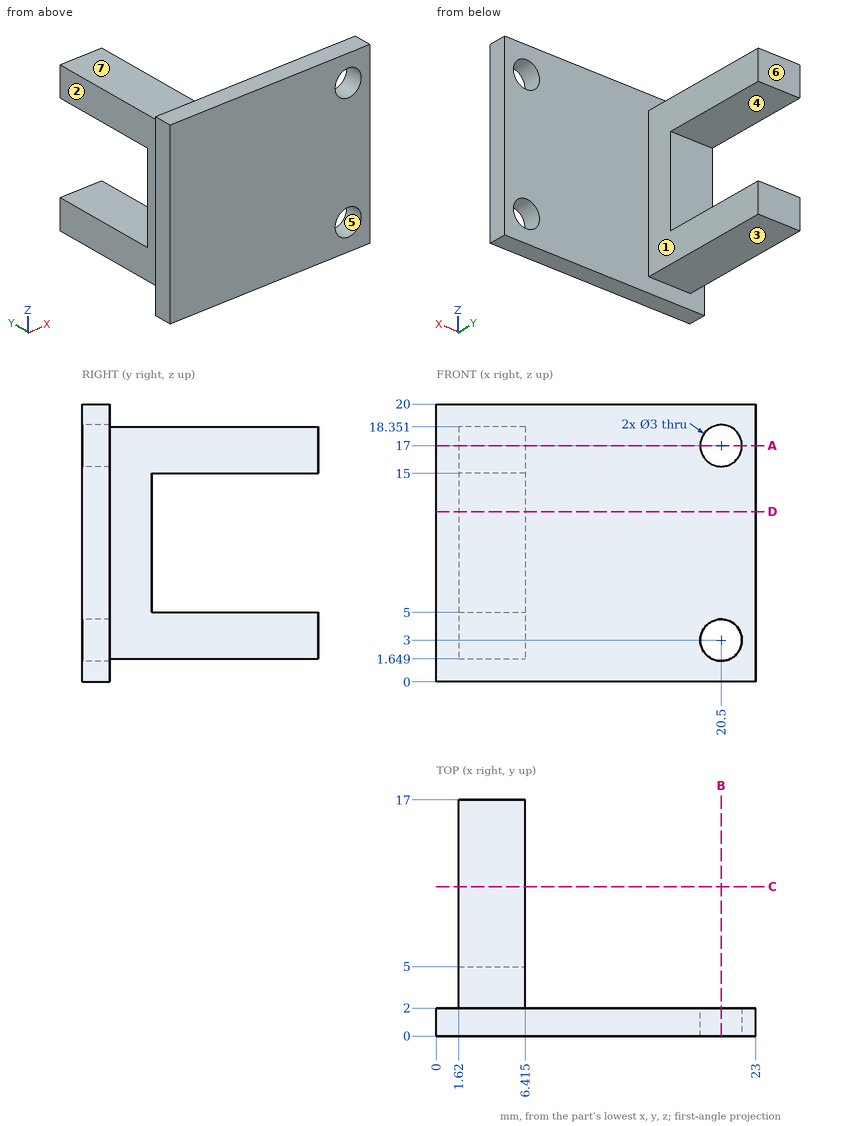
For this review, use the dimensioned drawing (mm, ordinates from the lowest corner) and the shaded views. A direction names the side the tool comes from. Round coordinates to 2 decimals unless told otherwise and drop trailing zeros. Write each loop counter-clockwise with the first axis right and the second up, starting at its lowest first coordinate (ties: lowest second). Pieces come first, ordered by that corner, then holes. Notation, with made-up numbers: (48.5, 14.5) - (103.5, 14.5) arc R28 cw to (103.5, 35.5) - close; hole circle Ø2 at (47.5, -40). An arc over 180 degrees is marked (long way). One line per item, written item: value. Start each with the question number.
1. To check wall thickness, follow L1, parallel to Z at x = 20.5, y = 1.05; L2, parallel to Z at x = 6, y = 7.25; L3, parallel to Z at x = 4.75, y = 2.75. State the ranges of each line that lie inside material, in increasing order. Write a range as from..to.
2. The part is to be moulded in two halves that separate along Z. For the marked faces 5, 6 and 7, say which applies: released by +Z, released by -Z, zero draft, split by the parting line, or undercut.
3. Consider section D-D on z = 12.25. Write out the cut boundary in (x, y) (1 decimal), and give its area (3 significant figures).
4. Consider section A-A on z = 17. Write out the cut boundary in (x, y) (1 decimal).
5. Consider section B-B on x = 20.5. Write out the cut boundary in (y, z).
6. Consider section C-C on y = 10.75. Write out the cut boundary in (x, z) (1 decimal).
7. Clearance check with flat-ended pins moving along their axes: P1, Ø1, axis at y = 12.5, z = 7, coming from the -X side; P2, Ø5.5, axis at x = 4.5, z = 10.5, coming from the +Y side; P3, Ø1.4, axis at x = 5, y = 12, coming from the +Z side; P4, Ø4, axis at x = 20.5, z = 17, coming from the +Y side. State where each tip first meets the part, or that it passes through.
8. Machinability: for the marked faces 1, 2, 3 and 4, which of the approach directions +Z, -Z, +X, -X, +Y, -Y give a long, thin tool a straight path to every point of the face, cutting with its end or side? Answer none if there is none.
Checks:
1. L1: z = 0..1.5, 4.5..15.5, 18.5..20
1. L2: z = 1.65..5, 15..18.35
1. L3: z = 1.65..18.35
2. face 5: undercut
2. face 6: zero draft
2. face 7: released by +Z
3. outline: (0, 0) - (23, 0) - (23, 2) - (6.4, 2) - (6.4, 5) - (1.6, 5) - (1.6, 2) - (0, 2) - close
3. area: 60.4 mm^2
4. outline: (0, 0) - (19, 0) - (19, 2) - (6.4, 2) - (6.4, 17) - (1.6, 17) - (1.6, 2) - (0, 2) - close; (22, 0) - (23, 0) - (23, 2) - (22, 2) - close
5. outline: (0, 0) - (2, 0) - (2, 1.5) - (0, 1.5) - close; (0, 4.5) - (2, 4.5) - (2, 15.5) - (0, 15.5) - close; (0, 18.5) - (2, 18.5) - (2, 20) - (0, 20) - close
6. outline: (1.6, 1.6) - (6.4, 1.6) - (6.4, 5) - (1.6, 5) - close; (1.6, 15) - (6.4, 15) - (6.4, 18.4) - (1.6, 18.4) - close
7. P1: passes through
7. P2: stops at y = 5
7. P3: stops at z = 18.35
7. P4: stops at y = 2
8. face 1: +Z, -Z, +X, +Y
8. face 2: +Z, -Z, -X, +Y
8. face 3: -Z, +X, -X, +Y
8. face 4: +X, -X, +Y
